from build123d import *

# Parameters (mm, degrees)
SKETCH_2_R          = 32.5
EXTRUDE_1_DEPTH     = 75
SKETCH_3_R          = 29
CUT_EXTRUDE_1_DEPTH = 142.5
SKETCH_4_W          = 65
SKETCH_4_H          = 75
CUT_EXTRUDE_2_DEPTH = 50
SKETCH_5_R          = 2
CUT_EXTRUDE_3_DEPTH = 50
FILLET_1_R          = 2
FILLET_2_R          = 2
FILLET_3_R          = 2


with BuildPart() as part:
    # 草圖2 → 填料-伸長1 (new body)
    with BuildSketch(Plane(origin=(0, 0, 0), x_dir=(1, 0, 0), z_dir=(0, 1, 0))):
        with Locations(Location((0, 0, 0), (0, 0, 270))):
            Circle(SKETCH_2_R)
    extrude(amount=EXTRUDE_1_DEPTH)

    # 草圖3 → 除料-伸長1 (cut, symmetric)
    with BuildSketch(Plane(origin=(0, 75, 0), x_dir=(1, 0, 0), z_dir=(0, 1, 0))):
        with Locations(Location((0, 0, 0), (0, 0, 270))):
            Circle(SKETCH_3_R)
    extrude(amount=CUT_EXTRUDE_1_DEPTH, both=True, mode=Mode.SUBTRACT)

    # 草圖4 → 除料-伸長2 (cut)
    with BuildSketch(Plane.XY):
        with Locations((0, 37.5)):
            Rectangle(SKETCH_4_W, SKETCH_4_H)
    extrude(amount=CUT_EXTRUDE_2_DEPTH, mode=Mode.SUBTRACT)

    # 草圖5 → 除料-伸長3 (cut)
    with BuildSketch(Plane.XY):
        with Locations((-4, 67)):
            Circle(SKETCH_5_R)
        with Locations((4, 67)):
            Circle(SKETCH_5_R)
        with Locations((12, 67)):
            Circle(SKETCH_5_R)
        with Locations((-12, 67)):
            Circle(SKETCH_5_R)
        with Locations((-12, 8)):
            Circle(SKETCH_5_R)
        with Locations((12, 8)):
            Circle(SKETCH_5_R)
        with Locations((4, 8)):
            Circle(SKETCH_5_R)
        with Locations((-4, 8)):
            Circle(SKETCH_5_R)
    extrude(amount=-CUT_EXTRUDE_3_DEPTH, mode=Mode.SUBTRACT)

    # 圓角1
    fillet_1_edges = [part.edges().sort_by_distance(p)[0] for p in [
        (-29, 37.5, 0),
        (29, 37.5, 0),
    ]]
    fillet(fillet_1_edges, radius=FILLET_1_R)

    # 圓角2
    fillet_2_edges = [part.edges().sort_by_distance(p)[0] for p in [
        (31.717708298, 75, 0),
        (0, 75, -29),
        (-31.717708298, 75, 0),
        (-29.567583368, 75, -0.540879629),
        (29.567583368, 75, -0.540879629),
    ]]
    fillet(fillet_2_edges, radius=FILLET_2_R)

    # 圓角3
    fillet_3_edges = [part.edges().sort_by_distance(p)[0] for p in [
        (-31.717708298, 0, 0),
        (31.717708298, 0, 0),
        (0, 0, -29),
        (-29.567583368, 0, -0.540879629),
        (29.567583368, 0, -0.540879629),
    ]]
    fillet(fillet_3_edges, radius=FILLET_3_R)


solid = part.part
The listing builds one solid part. Answer for the finished solid, in the listing's coordinates (mm). A direction names the side the tool comes from. Give positions to 0.01 mm unless a question says otherwise; leave off trailing zeros. Order: outer loops, then holes, each group sorted by start corner. A loop starts at its lowest first (then second) coordinate and runs counter-clockwise, first axis right, second up. Notation, with made-up numbers: (51.25, 79) -> (98.25, 79) arc R30 ccw to (98.25, 107) -> close; hole circle Ø4 at (23, -5.75). An arc over 180 degrees is marked (long way). Put each result on its own line as item: value.
Item 1: Given P1, Ø4, axis at x = -11.5, y = 58.5, coming from the -Z side; P2, Ø3, axis at y = 56.5, z = -10.5, coming from the -X side; P3, Ø5, axis at y = 21.5, z = -8.5, coming from the +X side; P4, Ø2.5, axis at x = 12, y = 8, coming from the -Z side, each flat-ended and moving along its own axis, determine where each tip first touches the part or whether it passes through.
Established:
P1: stops at z = -31.08
P2: stops at x = -31.23
P3: stops at x = 31.94
P4: passes through
Item 2: For a pull along X with two mould halves and no side action, classify faces 3 (the face through (5, 0, -31)), 4 (the face through (29.58, 38, -0.53)), 5 (the face through (0.715, 36.975, -32.492)) as released by +X, released by -X, zero draft, split by the parting line, or undercut.
Established:
face 3: zero draft
face 4: undercut
face 5: split by the parting line
Item 3: For faces 1 (the face through (-29.58, 38, -0.53)), 2 (the face through (-13.6, 6.8, -28.1)), determine the directions among +Z, -Z, +X, -X, +Y, -Y from which every point of the face is accessible in a straight line to the end or side of a thin tool.
Established:
face 1: +Z, +Y, -Y
face 2: +Z, -Z
Item 4: A cutting plane is placed at C-C on x = 4. Count the separate pieces of the cut face and the enclosed holes in it, plus the area to 3 significant figures.
Established:
separate pieces: 3
enclosed holes: 0
area: 235 mm^2
Item 5: Straight lines are drawn through the part: line 1 (X direction, y = 8, z = -29.4); line 2 (Y direction, x = -12, z = -28.85); line 3 (Y direction, x = 4, z = -30). For each, find the intervals that lie inside material, in ascending order.
Established:
line 1: x = -10 to -6, -2 to 2, 6 to 10
line 2: y = 0 to 6, 10 to 65, 69 to 75
line 3: y = 0.14 to 6, 10 to 65, 69 to 74.86
Item 6: A cutting plane is placed at A-A on y = 67. Give the vertices of the cut face in (x, z), plus the area to 3 significant figures.
Established:
outline: (-32.5, 0) arc R32.5 ccw to (-14, -29.33) -> (-14, -25.4) arc R29 cw to (-28.94, -1.87) arc R2 ccw to (-30.94, 0) -> close; (-10, -30.92) arc R32.5 ccw to (-6, -31.94) -> (-6, -28.37) arc R29 cw to (-10, -27.22) -> close; (-2, -32.44) arc R32.5 ccw to (2, -32.44) -> (2, -28.93) arc R29 cw to (-2, -28.93) -> close; (6, -31.94) arc R32.5 ccw to (10, -30.92) -> (10, -27.22) arc R29 cw to (6, -28.37) -> close; (14, -29.33) arc R32.5 ccw to (32.5, 0) -> (30.94, 0) arc R2 ccw to (28.94, -1.87) arc R29 cw to (14, -25.4) -> close
area: 278 mm^2
Item 7: A cutting plane is placed at B-B on y = 16. Give the vertices of the cut face in (x, z).
Established:
outline: (-32.5, 0) arc R32.5 ccw to (32.5, 0) -> (30.94, 0) arc R2 ccw to (28.94, -1.87) arc R29 cw to (-28.94, -1.87) arc R2 ccw to (-30.94, 0) -> close
